from build123d import *

# Parameters (mm, degrees)
SKETCH1_W                = 59
SKETCH1_H                = 34
SKETCH1_W_2              = 55
SKETCH1_H_2              = 28
BOSS_EXTRUDE1_DEPTH      = 25
SKETCH1_2_W              = 55
SKETCH1_2_H              = 28
BOSS_EXTRUDE2_DEPTH      = 2
SKETCH2_W                = 2
SKETCH2_H                = 34
CUT_EXTRUDE1_DEPTH       = 25
SKETCH5_W                = 2
SKETCH5_H                = 2
CUT_EXTRUDE4_DEPTH       = 51
SKETCH9_W                = 10
SKETCH9_H                = 10
CUT_EXTRUDE7_DEPTH       = 2.5
SKETCH10_W               = 10
SKETCH10_H               = 10
CUT_EXTRUDE8_DEPTH       = 2.5
SKETCH11_R               = 1
CUT_EXTRUDE9_DEPTH       = 12.5
CUT_EXTRUDE9_DEPTH_BACK  = 2.5
SKETCH12_R               = 1
CUT_EXTRUDE10_DEPTH      = 12.5
CUT_EXTRUDE10_DEPTH_BACK = 2.5


with BuildPart() as part:
    # Sketch1 → Boss-Extrude1 (new body)
    with BuildSketch(Plane(origin=(0, 0, 0), x_dir=(1, 0, 0), z_dir=(0, 1, 0))):
        with Locations((29.5, 17)):
            Rectangle(SKETCH1_W, SKETCH1_H)
        with Locations((29.5, 17)):
            Rectangle(SKETCH1_W_2, SKETCH1_H_2, mode=Mode.SUBTRACT)
    extrude(amount=BOSS_EXTRUDE1_DEPTH)

    # Sketch1_2 → Boss-Extrude2 (add)
    with BuildSketch(Plane(origin=(0, 0, 0), x_dir=(1, 0, 0), z_dir=(0, 1, 0))):
        with Locations((29.5, 17)):
            Rectangle(SKETCH1_2_W, SKETCH1_2_H)
    extrude(amount=BOSS_EXTRUDE2_DEPTH)

    # Sketch2 → Cut-Extrude1 (cut)
    with BuildSketch(Plane(origin=(0, 25, 0), x_dir=(1, 0, 0), z_dir=(0, 1, 0))):
        with Locations((58, 17)):
            Rectangle(SKETCH2_W, SKETCH2_H)
    extrude(amount=-CUT_EXTRUDE1_DEPTH, mode=Mode.SUBTRACT)

    # Sketch5 → Cut-Extrude4 (cut)
    with BuildSketch(Plane(origin=(57, 0, 0), x_dir=(0, 0, -1), z_dir=(1, 0, 0))):
        with Locations((2, 23)):
            Rectangle(SKETCH5_W, SKETCH5_H)
        with Locations((32, 23)):
            Rectangle(SKETCH5_W, SKETCH5_H)
    extrude(amount=-CUT_EXTRUDE4_DEPTH, mode=Mode.SUBTRACT)

    # Sketch9 → Cut-Extrude7 (cut)
    with BuildSketch(Plane(origin=(0, 0, -34), x_dir=(-1, 0, 0), z_dir=(0, 0, -1))):
        with Locations((-52, 13)):
            Rectangle(SKETCH9_W, SKETCH9_H)
    extrude(amount=-CUT_EXTRUDE7_DEPTH, mode=Mode.SUBTRACT)

    # Sketch10 → Cut-Extrude8 (cut)
    with BuildSketch(Plane.XY):
        with Locations((52, 13)):
            Rectangle(SKETCH10_W, SKETCH10_H)
    extrude(amount=-CUT_EXTRUDE8_DEPTH, mode=Mode.SUBTRACT)

    # Sketch11 → Cut-Extrude9 (cut, two sides)
    with BuildSketch(Plane(origin=(0, 18, 0), x_dir=(-1, 0, 0), z_dir=(0, -1, 0))) as cut_extrude9_sk:
        with Locations((-49, 1.3)):
            Circle(SKETCH11_R)
    extrude(amount=CUT_EXTRUDE9_DEPTH, mode=Mode.SUBTRACT)
    extrude(cut_extrude9_sk.sketch, amount=-CUT_EXTRUDE9_DEPTH_BACK, mode=Mode.SUBTRACT)

    # Sketch12 → Cut-Extrude10 (cut, two sides)
    with BuildSketch(Plane(origin=(0, 18, 0), x_dir=(-1, 0, 0), z_dir=(0, -1, 0))) as cut_extrude10_sk:
        with Locations((-48.8, 32.7)):
            Circle(SKETCH12_R)
    extrude(amount=CUT_EXTRUDE10_DEPTH, mode=Mode.SUBTRACT)
    extrude(cut_extrude10_sk.sketch, amount=-CUT_EXTRUDE10_DEPTH_BACK, mode=Mode.SUBTRACT)


solid = part.part
Can you work these out from the model? Positions are in its coordinate system, mm. A direction names the side the tool comes from. Coordinates: 2 decimals unless noted, no trailing zeros. Write each loop counter-clockwise with the first axis right and the second up, starting at its lowest first coordinate (ties: lowest second). Pieces come first, ordered by that corner, then holes.
Q1. Imagine slicing it at A-A, the plane y = 21.25. List the corners of the cut face in (x, z) for me, plus the area to 3 significant figures.
Results found:
outline: (0, -34) - (57, -34) - (57, -31) - (2, -31) - (2, -3) - (57, -3) - (57, 0) - (0, 0) - close
area: 398 mm2
Q2. Please list where these lines run through material, in increasing order: L1, parallel to Z at x = 15.5, y = 21; L2, parallel to X at y = 19.4, z = -1.3; L3, parallel to X at y = 7.3, z = -32.7.
Results found:
L1: z = -34 to -31, -3 to 0
L2: x = 0 to 48, 50 to 57
L3: x = 0 to 47.8, 49.8 to 57
Q3. If we mould it in two halves opening along X, with no side actions, what happens to faces 1 (the face through (49, 5.5, -1)), 2 (the face through (2, 13, -17)), 3 (the face through (32, 23, -33))? For each: +X half, -X half, draft (parallel to the pull), parting line (faces both ways), or undercut.
Results found:
face 1: undercut
face 2: +X half
face 3: draft
Q4. For P1, Ø3, axis at x = 50, y = 15, coming from the +Z side; P2, Ø2, axis at x = 29.5, z = -22.5, coming from the +Y side, each with a flat end and sliding along its axis, tell me the tip position at first contact or that it passes through.
Results found:
P1: stops at z = -2.5
P2: stops at y = 2
Q5. Imagine slicing it at D-D, the plane y = 15.5. List the corners of the cut face in (x, z) for me.
Results found:
outline: (0, -34) - (47, -34) - (47, -31.5) - (57, -31.5) - (57, -31) - (2, -31) - (2, -3) - (57, -3) - (57, -2.5) - (47, -2.5) - (47, 0) - (0, 0) - close
Q6. Imagine slicing it at B-B, the plane z = -14. List the corners of the cut face in (x, y) for me, plus the area to 3 significant figures.
Results found:
outline: (0, 0) - (57, 0) - (57, 2) - (2, 2) - (2, 25) - (0, 25) - close
area: 160 mm2
Q7. Imagine slicing it at C-C, the plane x = 9.5. List the corners of the cut face in (y, z) for me, plus the area to 3 significant figures.
Results found:
outline: (0, -34) - (25, -34) - (25, -31) - (24, -31) - (24, -33) - (22, -33) - (22, -31) - (2, -31) - (2, -3) - (22, -3) - (22, -1) - (24, -1) - (24, -3) - (25, -3) - (25, 0) - (0, 0) - close
area: 198 mm2
Q8. Which directions (+Z, -Z, +X, -X, +Y, -Y) give clear straight access to the entire face, cutting with the end or side of a thin tool? Please do faces 4 (the face through (29, 13, -31)), 5 (the face through (32, 24, -2)), 6 (the face through (52, 8, -33)).
Results found:
face 4: +X, +Y
face 5: +X
face 6: -Z, +X
